from build123d import *

# Parameters (mm, degrees)
CROQUIS1_W                          = 42
CROQUIS1_H                          = 42
SALIENTE_EXTRUIR1_DEPTH             = 39.4
CROQUIS2_W                          = 10.5
CROQUIS2_H                          = 16
SALIENTE_EXTRUIR2_DEPTH             = 6.5
CROQUIS3_R                          = 11
SALIENTE_EXTRUIR3_DEPTH             = 1.9
CROQUIS4_R                          = 2.45
SALIENTE_EXTRUIR4_DEPTH             = 20.4
CORTAR_EXTRUIR1_DEPTH               = 15
DI_METRO_DE_TALADRO_2_8_2_8_1_D     = 2.8
DI_METRO_DE_TALADRO_2_8_2_8_1_DEPTH = 3
CHAFL_N1_SIZE                       = 4
CROQUIS8_R                          = 2.5
CORTAR_EXTRUIR2_DEPTH               = 62.7


with BuildPart() as part:
    # Croquis1 → Saliente-Extruir1 (new body)
    with BuildSketch(Plane(origin=(0, 0, 0), x_dir=(-1, 0, 0), z_dir=(0, 0, -1))):
        with Locations((-21, 21)):
            Rectangle(CROQUIS1_W, CROQUIS1_H)
    extrude(amount=-SALIENTE_EXTRUIR1_DEPTH)

    # Croquis2 → Saliente-Extruir2 (add)
    with BuildSketch(Plane.ZY):
        with Locations((5.25, 21)):
            Rectangle(CROQUIS2_W, CROQUIS2_H)
    extrude(amount=SALIENTE_EXTRUIR2_DEPTH)

    # Croquis3 → Saliente-Extruir3 (add)
    with BuildSketch(Plane.XY.offset(39.4)):
        with Locations((21, 21)):
            Circle(CROQUIS3_R)
    extrude(amount=SALIENTE_EXTRUIR3_DEPTH)

    # Croquis4 → Saliente-Extruir4 (add)
    with BuildSketch(Plane.XY.offset(41.3)):
        with Locations((21, 21)):
            Circle(CROQUIS4_R)
    extrude(amount=SALIENTE_EXTRUIR4_DEPTH)

    # Croquis5 → Cortar-Extruir1 (cut)
    with BuildSketch(Plane.XY.offset(61.7)):
        with BuildLine():
            Line((22.99, 22.429125607), (22.99, 19.570874393))
            ThreePointArc((22.99, 19.570874393), (23.45, 21), (22.99, 22.429125607))
        make_face()
    extrude(amount=-CORTAR_EXTRUIR1_DEPTH, mode=Mode.SUBTRACT)

    # Diámetro de taladro Ø2.8 (2.8)1
    with Locations(Plane.XY.offset(39.4)):
        with Locations((36.5, 5.5), (5.5, 5.5), (36.5, 36.5), (5.5, 36.5)):
            Hole(DI_METRO_DE_TALADRO_2_8_2_8_1_D / 2, depth=DI_METRO_DE_TALADRO_2_8_2_8_1_DEPTH)

    # Chaflán1
    chafl_n1_edges = [part.edges().sort_by_distance(p)[0] for p in [
        (42, 0, 19.7),
        (42, 42, 19.7),
        (0, 42, 19.7),
        (0, 0, 19.7),
    ]]
    chamfer(chafl_n1_edges, length=CHAFL_N1_SIZE)

    # Croquis8 → Cortar-Extruir2 (cut, through all)
    with BuildSketch(Plane.XY.offset(61.7)):
        with Locations((21, 21)):
            Circle(CROQUIS8_R)
    extrude(amount=-CORTAR_EXTRUIR2_DEPTH, mode=Mode.SUBTRACT)


solid = part.part
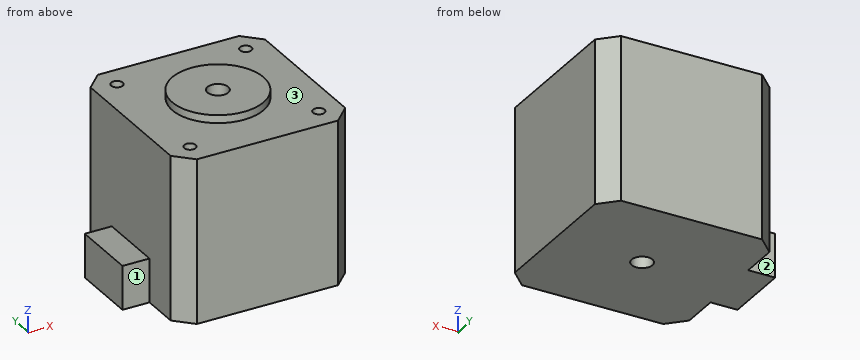
Verification items for the finished model (mm, model axes). Face numbers are marked on the shaded views. A direction names the side the tool comes from. Give positions to 0.01 mm unless a question says otherwise; leave off trailing zeros. Order: outer loops, then holes, each group sorted by start corner. A loop starts at its lowest first (then second) coordinate and runs counter-clockwise, first axis right, second up. Notation, with made-up numbers: M -16,50 L 42,50 A12 ccw 42,73 Z; hole C -18.5,13.25 d3. An arc over 180 degrees is marked long. Answer as a JSON object with one key per item and string values. Group by question number.
1) Scan lines: line 1 along Y through (x, z) = (21, 10.5); line 2 along Y through (x, z) = (5.5, 37.4); line 3 along Y through (x, z) = (5, 38). Record each from-to range of solid material in increasing order. Write a range as [from, to].
2) Cross-section at B-B (y = 21). Enter the section's corners in (x, z), then the cut area to 3 significant figures.
3) Access from +Z, -Z, +X, -X, +Y, -Y to the whole of each face (thin tool, end or side, straight path). Record for the marked faces 1, 2 and 3.
4) Cross-section at D-D (x = 5.5). Enter the section's corners in (y, z).
5) Depth check by flat-ended pin: pin 1 Ø2 at (x, z) = (-2.5, 5.5) entering from -Y; pin 2 Ø0.8 at (x, y) = (5, 5) entering from +Z; pin 3 Ø12 at (x, y) = (15, 8) entering from +Z; pin 4 Ø3 at (y, z) = (16.5, 27.5) entering from -X. Enter the tip coordinate at first touch or a pass-through.
6) Cross-section at C-C (z = 29). Enter the section's corners in (x, y), then the cut area to 3 significant figures.
7) Cross-section at A-A (x = 21). Enter the section's corners in (y, z), then the cut area to 3 significant figures.
Result sheet:
{
 "1": {"line 1": "y = [0, 18.5], [23.5, 42]", "line 2": "y = [0, 4.1], [6.9, 35.1], [37.9, 42]", "line 3": "y = [0, 4.19], [6.81, 35.19], [37.81, 42]"},
 "2": {"outline": "M -6.5,0 L 18.5,0 L 18.5,41.3 L 10,41.3 L 10,39.4 L 0,39.4 L 0,10.5 L -6.5,10.5 Z; M 23.5,0 L 42,0 L 42,39.4 L 32,39.4 L 32,41.3 L 23.5,41.3 Z", "area": "1,560 mm2"},
 "3": {"face 1": "+Z, -Z, -X, -Y", "face 2": "+Z, -Z, -X, +Y", "face 3": "+Z"},
 "4": {"outline": "M 0,0 L 42,0 L 42,39.4 L 37.9,39.4 L 37.9,36.4 L 35.1,36.4 L 35.1,39.4 L 6.9,39.4 L 6.9,36.4 L 4.1,36.4 L 4.1,39.4 L 0,39.4 Z"},
 "5": {"pin 1": "stops at y = 13", "pin 2": "stops at z = 36.4", "pin 3": "stops at z = 41.3", "pin 4": "stops at x = 0"},
 "6": {"outline": "M 0,4 L 4,0 L 38,0 L 42,4 L 42,38 L 38,42 L 4,42 L 0,38 Z; hole C 21,21 d5", "area": "1,710 mm2"},
 "7": {"outline": "M 0,0 L 18.5,0 L 18.5,41.3 L 10,41.3 L 10,39.4 L 0,39.4 Z; M 23.5,0 L 42,0 L 42,39.4 L 32,39.4 L 32,41.3 L 23.5,41.3 Z", "area": "1,490 mm2"}
}
